Can you work these out from the model? Positions are in its coordinate system, mm. Face numbers are marked on the shaded views. A direction names the side the tool comes from. Give positions to 0.01 mm unless a question says otherwise; leave off trailing zeros. Loops run counter-clockwise (first coordinate to the right, second up) from the corner with the lowest first, then second, coordinate; pieces in that order, holes last. Notation, with made-up numbers: (-23, 6) - (30, 6) arc R14 cw to (30, 14) - close; hole circle Ø7 at (-16, 68). An arc over 180 degrees is marked (long way). Answer as a JSON object with one key per item and string values. Group by question number.
Item 1: Which directions (+Z, -Z, +X, -X, +Y, -Y) give clear straight access to the entire face, cutting with the end or side of a thin tool? Please do the marked faces 1 and 2.
Item 2: Suppose I cut it at D-D on x = -23.5. Write out the boundary of the cut face in (y, z).
Item 3: Will these pins go through, and if not, where does the flat tip stop? pin 1 (3.5 mm diameter, centred on x = 28, y = 17.5, fed in from -Z); pin 2 (7.5 mm diameter, centred on x = -7.16, y = 0, fed in from -Z); pin 3 (1.6 mm diameter, centred on y = -24.5, z = 1, fed in from -X); pin 4 (8.5 mm diameter, centred on x = -9.5, y = 1.5, fed in from -Z).
Item 4: Suppose I cut it at C-C on y = 0. Write out the boundary of the cut face in (x, z).
Item 5: Suppose I cut it at A-A on x = 28. Write out the boundary of the cut face in (y, z).
Item 6: Suppose I cut it at B-B on z = 3.25. Write out the boundary of the cut face in (x, y).
Item 7: Thinking about a two-plate mould opening in Y: for the marked faces 3, 4 and 5, which applies, pulls with the +Y half, pulls with the -Y half, needs draft (parallel to the pull), parting line crosses it, or undercut?
Item 8: Please list where these lines run through material, in increasing order: L1, parallel to Y at x = 28, z = 2.5; L2, parallel to Y at x = 22.5, z = 1.75; L3, parallel to Z at x = 16, y = 21.5.
from build123d import *

# Parameters (mm, degrees)
F0_W      = 80
F0_H      = 60
F1_DEPTH  = 14
F2_W      = 80
F2_H      = 20
F3_DEPTH  = 2
F4_W      = 40
F4_H      = 20
F4_H_2    = 40
F5_DEPTH  = 2
F6_SIZE   = 10
F7_R      = 3.25
F8_DEPTH  = 25
F9_R      = 5.25
F10_DEPTH = 6.5
F12_D     = 4.2
F13_SIZE  = 1


with BuildPart() as f1:
    # F0 (on Top) → F1 (new body)
    with BuildSketch(Plane.XY):
        Rectangle(F0_W, F0_H)
    extrude(amount=F1_DEPTH)

    # F2 (on face) → F3 (cut)
    with BuildSketch(Plane(origin=(0, 0, 0), x_dir=(1, 0, 0), z_dir=(0, 0, -1))):
        Rectangle(F2_W, F2_H)
    extrude(amount=-F3_DEPTH, mode=Mode.SUBTRACT)

    # F4 (on face) → F5 (cut)
    with BuildSketch(Plane(origin=(0, 0, 0), x_dir=(1, 0, 0), z_dir=(0, 0, -1))):
        with Locations((0, 20)):
            Rectangle(F4_W, F4_H)
        with Locations((0, -10)):
            Rectangle(F4_W, F4_H_2)
    extrude(amount=-F5_DEPTH, mode=Mode.SUBTRACT)

    # F6
    f6_edges = [f1.edges().sort_by_distance(p)[0] for p in [
        (-40, 30, 7),
        (-40, -30, 7),
    ]]
    chamfer(f6_edges, length=F6_SIZE)

    # F7 (on face) → F8 (cut)
    with BuildSketch(Plane.XY.offset(14)):
        with Locations((-7.1571292716, 0)):
            Circle(F7_R)
    extrude(amount=-F8_DEPTH, mode=Mode.SUBTRACT)

    # F9 (on face) → F10 (cut)
    with BuildSketch(Plane(origin=(0, 0, 2), x_dir=(1, 0, 0), z_dir=(0, 0, -1))):
        with Locations((-7.1571292716, 0)):
            Circle(F9_R)
    extrude(amount=-F10_DEPTH, mode=Mode.SUBTRACT)

    # F12 (through all)
    with Locations(Plane.XY.offset(14)):
        with Locations((28, 17.5), (28, -17.5)):
            Hole(F12_D / 2)

    # F13
    f13_edges = [f1.edges().sort_by_distance(p)[0] for p in [
        (-40, 0, 14),
        (-35, 25, 14),
        (-35, -25, 14),
        (5, 30, 14),
        (5, -30, 14),
        (40, 0, 14),
        (25.9, -17.5, 14),
        (-10.407129, 0, 14),
        (25.9, 17.5, 14),
    ]]
    chamfer(f13_edges, length=F13_SIZE)


solid = f1.part
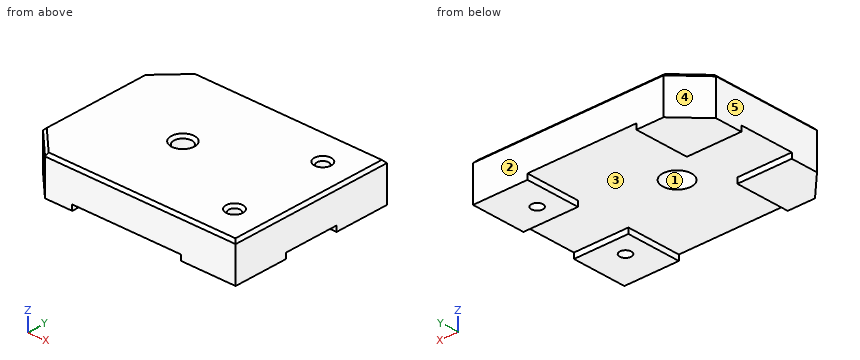
Worked out:
{
 "1": {"face 1": "-Z", "face 2": "+Z, -Z, +X, -X, +Y"},
 "2": {"outline": "(-30, 0) - (-10, 0) - (-10, 2) - (10, 2) - (10, 0) - (30, 0) - (30, 13) - (29, 14) - (-29, 14) - (-30, 13) - close"},
 "3": {"pin 1": "passes through", "pin 2": "stops at z = 8.5", "pin 3": "stops at x = -36.3", "pin 4": "stops at z = 2"},
 "4": {"outline": "(-40, 2) - (-12.41, 2) - (-12.41, 8.5) - (-10.41, 8.5) - (-10.41, 13) - (-11.41, 14) - (-39, 14) - (-40, 13) - close; (-3.91, 8.5) - (-1.91, 8.5) - (-1.91, 2) - (40, 2) - (40, 13) - (39, 14) - (-2.91, 14) - (-3.91, 13) - close"},
 "5": {"outline": "(-30, 0) - (-19.6, 0) - (-19.6, 13) - (-20.6, 14) - (-29, 14) - (-30, 13) - close; (-15.4, 0) - (-10, 0) - (-10, 2) - (10, 2) - (10, 0) - (15.4, 0) - (15.4, 13) - (14.4, 14) - (-14.4, 14) - (-15.4, 13) - close; (19.6, 0) - (30, 0) - (30, 13) - (29, 14) - (20.6, 14) - (19.6, 13) - close"},
 "6": {"outline": "(-40, -20) - (-30, -30) - (40, -30) - (40, 30) - (-30, 30) - (-40, 20) - close; hole circle Ø10.5 at (-7.16, 0); hole circle Ø4.2 at (28, -17.5); hole circle Ø4.2 at (28, 17.5)"},
 "7": {"face 3": "undercut", "face 4": "pulls with the +Y half", "face 5": "needs draft"},
 "8": {"L1": "y = -30 to -19.6, -15.4 to 15.4, 19.6 to 30", "L2": "y = -30 to -10, 10 to 30", "L3": "z = 2 to 14"}
}
